```python
from build123d import *

# Parameters (mm, degrees)
SKETCH1_R                            = 2.5
BOSS_EXTRUDE1_DEPTH                  = 30
SKETCH1_3_R                          = 2.5
CUT_EXTRUDE1_DEPTH                   = 10.25
F_6_5_6_5_DIAMETER_HOLE1_D           = 6.5
F_6_5_6_5_DIAMETER_HOLE1_CSINK_D     = 7
F_6_5_6_5_DIAMETER_HOLE1_CSINK_ANGLE = 90
FILLET1_R                            = 5


with BuildPart() as part:
    # Sketch1 → Boss-Extrude1 (new, symmetric)
    with BuildSketch(Plane(origin=(0, 0, 0), x_dir=(1, 0, 0), z_dir=(0, 1, 0))):
        with BuildLine():
            Line((4.582575695, 0), (4.582575695, 2))
            ThreePointArc((4.582575695, 2), (-5, 0), (4.582575695, -2))
            Line((4.582575695, -2), (30, -2))
            Line((30, -2), (30, 0))
            Line((30, 0), (4.582575695, 0))
        make_face()
        with Locations(Location((0, 0, 0), (0, 0, 270))):
            Circle(SKETCH1_R, mode=Mode.SUBTRACT)
    extrude(amount=BOSS_EXTRUDE1_DEPTH, both=True)

    # Sketch1_3 → Cut-Extrude1 (cut, symmetric)
    with BuildSketch(Plane(origin=(0, 0, 0), x_dir=(1, 0, 0), z_dir=(0, 1, 0))):
        with BuildLine():
            Line((4.582575695, -2), (5.5, -2))
            Line((5.5, -2), (5.5, 0))
            Line((5.5, 0), (4.582575695, 0))
            Line((4.582575695, 0), (4.582575695, 2))
            ThreePointArc((4.582575695, 2), (-5, 0), (4.582575695, -2))
        make_face()
        with Locations(Location((0, 0, 0), (0, 0, 270))):
            Circle(SKETCH1_3_R, mode=Mode.SUBTRACT)
    extrude(amount=CUT_EXTRUDE1_DEPTH, both=True, mode=Mode.SUBTRACT)

    # 6.5 _6.5_ Diameter Hole1 (through all)
    with Locations(Plane(origin=(0, 0, 0), x_dir=(-1, 0, 0), z_dir=(0, 0, -1))):
        with Locations((-20, -20), (-20, 0), (-20, 20)):
            CounterSinkHole(F_6_5_6_5_DIAMETER_HOLE1_D / 2, F_6_5_6_5_DIAMETER_HOLE1_CSINK_D / 2, counter_sink_angle=F_6_5_6_5_DIAMETER_HOLE1_CSINK_ANGLE)

    # Fillet1
    fillet1_edges = [part.edges().sort_by_distance(p)[0] for p in [
        (30, 30, 1),
        (30, -30, 1),
    ]]
    fillet(fillet1_edges, radius=FILLET1_R)


solid = part.part
```
The listing builds one solid part. Answer for the finished solid, in the listing's coordinates (mm). A direction names the side the tool comes from. Round coordinates to 2 decimals unless told otherwise and drop trailing zeros. Loops run counter-clockwise (first coordinate to the right, second up) from the corner with the lowest first, then second, coordinate; pieces in that order, holes last.
Q1. Section D-D, the plane z = -1.25 is taken. Determine the outline of the cut face in (x, y).
Q2. Section A-A, the plane y = -20 is taken. Determine the outline of the cut face in (x, z).
Q3. Given pin 1 Ø6 at (x, y) = (8, 2) entering from -Z; pin 2 Ø7.5 at (x, y) = (19.5, 4.5) entering from +Z; pin 3 Ø6 at (x, y) = (20, 20) entering from -Z (3 decimals); pin 4 Ø1.6 at (y, z) = (-3.5, 1) entering from -X, each flat-ended and moving along its own axis, determine where each tip first touches the part or whether it passes through.
Q4. Which of the six approach directions +Z, -Z, +X, -X, +Y, -Y give full straight-line access (tool end or side, diameter ignored) to faces 1 (the face through (5.5, 0, 1)), 2 (the face through (28, 29, 1)), 3 (the face through (14, 0, 2)), 4 (the face through (4.583, -20, -1))?
Q5. Find the intervals of material crossed by line 1 (X direction, y = 0, z = 0.6); line 2 (Y direction, x = -2, z = -3.5); line 3 (Z direction, x = 24, y = -20), in increasing order.
Q6. Section C-C, the plane y = 0 is taken. Determine the outline of the cut face in (x, z), then the cut area to 3 significant figures.
Q7. For a pull along X with two mould halves and no side action, classify faces 5 (the face through (17.605, -17.803, 1.137)), 6 (the face through (3, -10.25, 0)), 7 (the face through (30, 0, 1)) as released by +X, released by -X, zero draft, split by the parting line, or undercut.
Q8. Section B-B, the plane x = 0 is taken. Determine the outline of the cut face in (y, z), then the cut area to 4 significant figures.
Completed:
1. outline: (-4.84, -30) - (-2.17, -30) - (-2.17, -10.25) - (-4.84, -10.25) - close; (-4.84, 10.25) - (-2.17, 10.25) - (-2.17, 30) - (-4.84, 30) - close; (2.17, -30) - (4.58, -30) - (4.58, -10.25) - (2.17, -10.25) - close; (2.17, 10.25) - (4.58, 10.25) - (4.58, 30) - (2.17, 30) - close
2. outline: (4.58, -2) - (4.58, 0) - (16.5, 0) - (16.75, 0.25) - (16.75, 2) - (4.58, 2) arc R5 ccw (long way) to start; (23.25, 0.25) - (23.5, 0) - (30, 0) - (30, 2) - (23.25, 2) - close; hole circle Ø5 at (0, 0)
3. pin 1: stops at z = 0
3. pin 2: stops at z = 2
3. pin 3: passes through
3. pin 4: stops at x = 5.5
4. face 1: +Z, -Z, -X
4. face 2: +Z, -Z, +X, +Y
4. face 3: +Z, +X, +Y, -Y
4. face 4: -Z, +X, +Y, -Y
5. line 1: x = 5.5 to 16.75, 23.25 to 30
5. line 2: y = -30 to -10.25, 10.25 to 30
5. line 3: z = 0 to 2
6. outline: (5.5, 0) - (16.5, 0) - (16.75, 0.25) - (16.75, 2) - (5.5, 2) - close; (23.25, 0.25) - (23.5, 0) - (30, 0) - (30, 2) - (23.25, 2) - close
6. area: 35.9 mm2
7. face 5: undercut
7. face 6: zero draft
7. face 7: released by +X
8. outline: (-30, -5) - (-10.25, -5) - (-10.25, -2.5) - (-30, -2.5) - close; (-30, 2.5) - (-10.25, 2.5) - (-10.25, 5) - (-30, 5) - close; (10.25, -5) - (30, -5) - (30, -2.5) - (10.25, -2.5) - close; (10.25, 2.5) - (30, 2.5) - (30, 5) - (10.25, 5) - close
8. area: 197.5 mm2
